Here's how the part is built. I have some questions about the finished solid (model axes, mm). A direction names the side the tool comes from. Coordinates: 2 decimals unless noted, no trailing zeros. Write each loop counter-clockwise with the first axis right and the second up, starting at its lowest first coordinate (ties: lowest second). Pieces come first, ordered by that corner, then holes.
Item 1: I want a section at A-A (z = 1.95). Please give me the cut outline in (x, y).
Item 2: For faces 1 (the face through (22, 24, 1)), 2 (the face through (-23, -30.725, 1)), 3 (the face through (22, -46, 1)), which set-ups out of +Z, -Z, +X, -X, +Y, -Y let a thin tool reach every point of the face, with its end or its side?
Item 3: I want a section at B-B (y = -37). Please give me the cut outline in (x, z), and give its area (3 significant figures).
Item 4: Please list where these lines run through material, in increasing order: line 1 (Y direction, x = 14.5, z = 0.1); line 2 (Y direction, x = -15, z = 0.45); line 3 (X direction, y = 8, z = 2.5).
Item 5: I'm going to push flat-ended pins straight in: P1, Ø1.5, axis at y = -44, z = 1, coming from the +X side; P2, Ø0.9, axis at y = -51.5, z = 1, coming from the -X side; P3, Ø1.5, axis at x = -23, z = 2, coming from the +Y side. Where does each tip first touch, or does it pass through?
Item 6: If we mould it in two halves opening along X, with no side actions, what happens to faces 4 (the face through (-11.79, 9.32, 1.48)), 5 (the face through (-22, 24, 1)), 6 (the face through (-24, 9.275, 1)), 7 (the face through (-15.252, -29.507, 1.479))? For each: pulls with the +X half, pulls with the -X half, needs draft (parallel to the pull), parting line crosses it, or undercut.
from build123d import *

# Parameters (mm, degrees)
SKETCH1_R           = 2.5
BOSS_EXTRUDE1_DEPTH = 3


with BuildPart() as part:
    # Sketch1 → Boss-Extrude1 (new body)
    with BuildSketch(Plane.XY):
        Polygon((-25, 9.275362319), (-22, 9.275362319), (-22, 39.275362319), (22, 39.275362319), (22, 9.275362319), (25, 9.275362319), (25, -30.724637681), (22, -30.724637681), (22, -60.724637681), (-22, -60.724637681), (-22, -30.724637681), (-25, -30.724637681), align=None)
        with Locations((15.558956534, 10.275362319)):
            Circle(SKETCH1_R, mode=Mode.SUBTRACT)
        with Locations((-14.098613638, 10.275362319)):
            Circle(SKETCH1_R, mode=Mode.SUBTRACT)
        with Locations(Location((15.558956534, -31.724637681, 0), (0, 0, 180))):
            Circle(SKETCH1_R, mode=Mode.SUBTRACT)
        with Locations(Location((-14.098613638, -31.724637681, 0), (0, 0, 180))):
            Circle(SKETCH1_R, mode=Mode.SUBTRACT)
    extrude(amount=BOSS_EXTRUDE1_DEPTH)


solid = part.part
Answer:
1. outline: (-25, -30.72) - (-22, -30.72) - (-22, -60.72) - (22, -60.72) - (22, -30.72) - (25, -30.72) - (25, 9.28) - (22, 9.28) - (22, 39.28) - (-22, 39.28) - (-22, 9.28) - (-25, 9.28) - close; hole circle Ø5 at (-14.1, -31.72); hole circle Ø5 at (-14.1, 10.28); hole circle Ø5 at (15.56, -31.72); hole circle Ø5 at (15.56, 10.28)
2. face 1: +Z, -Z, +X, +Y
2. face 2: +Z, -Z, -X, -Y
2. face 3: +Z, -Z, +X, -Y
3. outline: (-22, 0) - (22, 0) - (22, 3) - (-22, 3) - close
3. area: 132 mm2
4. line 1: y = -60.72 to -33.99, -29.46 to 8.01, 12.54 to 39.28
4. line 2: y = -60.72 to -34.06, -29.39 to 7.94, 12.61 to 39.28
4. line 3: x = -25 to -15.13, -13.06 to 14.52, 16.59 to 25
5. P1: stops at x = 22
5. P2: stops at x = -22
5. P3: stops at y = 9.28
6. face 4: undercut
6. face 5: pulls with the -X half
6. face 6: needs draft
6. face 7: undercut
